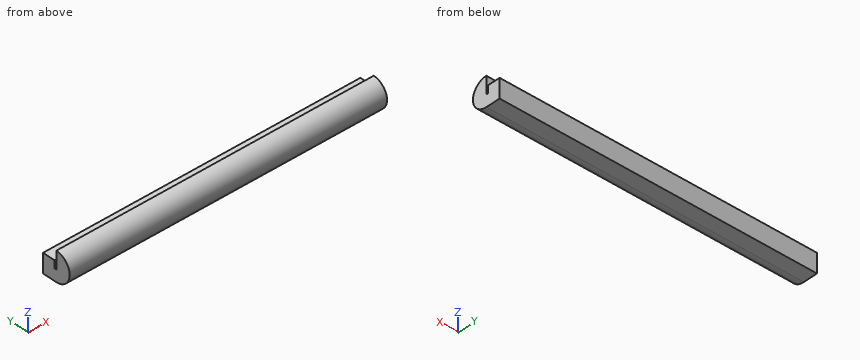
```python
from build123d import *

# Parameters (mm, degrees)
F1_DEPTH = 279.4


with BuildPart() as f1:
    # F0 (on Right) → F1 (new body)
    with BuildSketch(Plane.YZ):
        with BuildLine():
            Line((0, -15.190765), (0, 0))
            ThreePointArc((0, 0), (-12.7, -12.7), (0, -25.4))
            Line((0, -25.4), (0, -15.190765))
        make_face()
        Polygon((1.590656, -15.190765), (0, -15.190765), (0, -25.4), (12.7, -25.4), (12.7, -8.669076), (1.590656, -8.669076), align=None)
    extrude(amount=F1_DEPTH)


solid = f1.part
```
Work out the finished part from the listing and answer in its coordinate system (mm). Give positions to 0.01 mm unless a question says otherwise; leave off trailing zeros. Loops run counter-clockwise (first coordinate to the right, second up) from the corner with the lowest first, then second, coordinate; pieces in that order, holes last. Notation, with made-up numbers: (11, 25) -> (22, 25) arc R20 cw to (22, 64) -> close; hole circle Ø5 at (-6, 33.25). An arc over 180 degrees is marked (long way). One line per question, with ' | ' between items. Start each with the question number.
1) Straight lines are drawn through the part: L1, parallel to Z at x = 253, y = 6.5; L2, parallel to Z at x = 25, y = 1.25; L3, parallel to Y at x = 22, z = -13.75. For each, find the intervals that lie inside material, in ascending order.
2) Section B-B, the plane x = 42 is taken. Determine the outline of the cut face in (y, z), then the cut area to 3 significant figures.
3) Each of these flat-tipped pins is pushed along its axis until it touches: pin 1 (1.5 mm diameter, centred on x = 194.5, z = -19.5, fed in from -Y); pin 2 (8 mm diameter, centred on x = 173.5, z = -19, fed in from -Y); pin 3 (2 mm diameter, centred on y = 0.5, z = -8.5, fed in from -X); pin 4 (4 mm diameter, centred on x = 31.5, y = -7.5, fed in from -Z). Where does it stop, or does it pass through?
4) Section A-A, the plane z = -12.7 is taken. Determine the outline of the cut face in (x, y).
5) Section C-C, the plane y = 7 is taken. Determine the outline of the cut face in (x, z), then the cut area to 3 significant figures.
6) Section D-D, the plane y = -8 is taken. Determine the outline of the cut face in (x, z), then the cut area to 3 significant figures.
Resolved:
1) L1: -25.4 to -8.67 | L2: -25.4 to -15.19 | L3: -12.66 to 0, 1.59 to 12.7
2) outline: (0, -25.4) -> (12.7, -25.4) -> (12.7, -8.67) -> (1.59, -8.67) -> (1.59, -15.19) -> (0, -15.19) -> (0, 0) arc R12.7 ccw to start | area: 455 mm2
3) pin 1: y = -11.17 | pin 2: y = -12.49 | pin 3: x = 0 | pin 4: z = -24.15
4) outline: (0, -12.7) -> (279.4, -12.7) -> (279.4, 0) -> (0, 0) -> close; (0, 1.59) -> (279.4, 1.59) -> (279.4, 12.7) -> (0, 12.7) -> close
5) outline: (0, -25.4) -> (279.4, -25.4) -> (279.4, -8.67) -> (0, -8.67) -> close | area: 4,670 mm2
6) outline: (0, -22.56) -> (279.4, -22.56) -> (279.4, -2.84) -> (0, -2.84) -> close | area: 5,510 mm2
